Source: CAD feature listing. Evaluate the final solid. Frame: model axes, mm. A direction names the side the tool comes from. Round coordinates to 2 decimals unless told otherwise and drop trailing zeros. Write each loop counter-clockwise with the first axis right and the second up, starting at its lowest first coordinate (ties: lowest second). Pieces come first, ordered by that corner, then holes.
```python
from build123d import *

# Parameters (mm, degrees)
SKETCH1_R                 = 50
BOSS_EXTRUDE1_DEPTH       = 10
SKETCH2_R                 = 5
CUT_EXTRUDE1_DEPTH        = 10
SKETCH6_W                 = 5
SKETCH6_H                 = 35
BOSS_EXTRUDE4_DEPTH       = 20
SKETCH7_W                 = 5
SKETCH7_H                 = 20
BOSS_EXTRUDE5_DEPTH       = 40
F_2_0MM_DOWEL_HOLE1_D     = 2
F_2_0MM_DOWEL_HOLE1_DEPTH = 10
F_2_0MM_DOWEL_HOLE1_TIP   = 0.600860619
SKETCH12_R                = 3.75
BOSS_EXTRUDE6_DEPTH       = 10


with BuildPart() as part:
    # Sketch1 → Boss-Extrude1 (new body)
    with BuildSketch(Plane(origin=(0, 0, 0), x_dir=(1, 0, 0), z_dir=(0, 1, 0))):
        with Locations(Location((0, 0, 0), (0, 0, 270))):
            Circle(SKETCH1_R)
    extrude(amount=BOSS_EXTRUDE1_DEPTH)

    # Sketch2 → Cut-Extrude1 (cut)
    with BuildSketch(Plane(origin=(0, 10, 0), x_dir=(1, 0, 0), z_dir=(0, 1, 0))):
        with Locations(Location((0, 0, 0), (0, 0, 270))):
            Circle(SKETCH2_R)
    extrude(amount=-CUT_EXTRUDE1_DEPTH, mode=Mode.SUBTRACT)

    # Sketch6 → Boss-Extrude4 (add)
    with BuildSketch(Plane(origin=(0, 10, 0), x_dir=(1, 0, 0), z_dir=(0, 1, 0))):
        with Locations((12.5, -2.5)):
            Rectangle(SKETCH6_W, SKETCH6_H)
        with Locations((-32.5, -2.5)):
            Rectangle(SKETCH6_W, SKETCH6_H)
    extrude(amount=BOSS_EXTRUDE4_DEPTH)

    # Sketch7 → Boss-Extrude5 (add)
    with BuildSketch(Plane(origin=(-30, 0, 0), x_dir=(0, 0, -1), z_dir=(1, 0, 0))):
        with Locations((-17.5, 20)):
            Rectangle(SKETCH7_W, SKETCH7_H)
    extrude(amount=BOSS_EXTRUDE5_DEPTH)

    # 2.0mm Dowel Hole1
    with Locations(Plane(origin=(0, 0, -15), x_dir=(-1, 0, 0), z_dir=(0, 0, -1))):
        with Locations((-12.5, 24.873818091), (-12.5, 14.873818091)):
            Hole(F_2_0MM_DOWEL_HOLE1_D / 2, depth=F_2_0MM_DOWEL_HOLE1_DEPTH)
            with Locations((0, 0, -(F_2_0MM_DOWEL_HOLE1_DEPTH + F_2_0MM_DOWEL_HOLE1_TIP / 2))):  # 118° drill point
                Cone(0, F_2_0MM_DOWEL_HOLE1_D / 2, F_2_0MM_DOWEL_HOLE1_TIP, mode=Mode.SUBTRACT)

    # Sketch12 → Boss-Extrude6 (add)
    with BuildSketch(Plane.XY.offset(20)):
        with Locations(Location((0, 20, 0), (0, 0, 180))):
            Circle(SKETCH12_R)
    extrude(amount=BOSS_EXTRUDE6_DEPTH)


solid = part.part
```
Q1. Mould query, pull axis Z, two halves, no side actions, for faces 4 (the face through (12, 20, -15)), 5 (the face through (-4.88, 5.07, -1.08)), 6 (the face through (-35, 20, 3)). Classes: pulls with the +Z half, pulls with the -Z half, needs draft (parallel to the pull), parting line crosses it, or undercut.
Q2. Section query A-A, the plane x = 0. Output: boundary loops of the cut face in (y, z).
Q3. Section query C-C, the plane y = 20. Output: boundary loops of the cut face in (x, z).
Q4. Set-up query: faces 1 (the face through (0, 20, 30)), 2 (the face through (15, 20, 3)), 3 (the face through (-30, 20, 0)). Return all of +Z, -Z, +X, -X, +Y, -Y with unobstructed straight access to the full face (end or side cutting, diameter ignored); none if empty.
Q5. Section query B-B, the plane z = 0. Output: boundary loops of the cut face in (x, y), and give its area (3 significant figures).
Q6. Pin query (flat end, axial travel): P1, Ø2, axis at x = -32.5, y = 22, coming from the +Z side; P2, Ø1, axis at y = 23.5, z = -3, coming from the +X side; P3, Ø10, axis at y = 15.5, z = -2.5, coming from the -X side. Return the tip coordinate at first contact, or that it passes through.
Q7. Section query D-D, the plane z = -12. Output: boundary loops of the cut face in (x, y).
Q8. Line query: line 1 (Y direction, x = 12.5, z = -10.5); line 2 (X direction, y = 28.5, z = 5.5); line 3 (X direction, y = 7, z = 0). Output: solid intervals per line, ascending.
Filled in:
1. face 4: pulls with the -Z half
1. face 5: undercut
1. face 6: needs draft
2. outline: (0, -50) - (10, -50) - (10, -5) - (0, -5) - close; (0, 5) - (10, 5) - (10, 15) - (30, 15) - (30, 20) - (23.75, 20) - (23.75, 30) - (16.25, 30) - (16.25, 20) - (10, 20) - (10, 50) - (0, 50) - close
3. outline: (-35, -15) - (-30, -15) - (-30, 15) - (10, 15) - (10, -15) - (15, -15) - (15, 20) - (3.75, 20) - (3.75, 30) - (-3.75, 30) - (-3.75, 20) - (-35, 20) - close
4. face 1: +Z, +X, -X, +Y
4. face 2: +Z, -Z, +X, +Y
4. face 3: -Z, +Y
5. outline: (-50, 0) - (-5, 0) - (-5, 10) - (-30, 10) - (-30, 30) - (-35, 30) - (-35, 10) - (-50, 10) - close; (5, 0) - (50, 0) - (50, 10) - (15, 10) - (15, 30) - (10, 30) - (10, 10) - (5, 10) - close
5. area: 1,100 mm2
6. P1: stops at z = 20
6. P2: stops at x = 15
6. P3: stops at x = -35
7. outline: (-48.54, 0) - (48.54, 0) - (48.54, 10) - (15, 10) - (15, 30) - (10, 30) - (10, 10) - (-30, 10) - (-30, 30) - (-35, 30) - (-35, 10) - (-48.54, 10) - close; hole circle Ø2 at (12.5, 14.87); hole circle Ø2 at (12.5, 24.87)
8. line 1: y = 0 to 13.87, 15.87 to 23.87, 25.87 to 30
8. line 2: x = -35 to -30, 10 to 15
8. line 3: x = -50 to -5, 5 to 50
